```python
from build123d import *

# Parameters (mm, degrees)
SKETCH2_W           = 62.5
SKETCH2_H           = 62.5
CUT_EXTRUDE1_DEPTH  = 50
BOSS_EXTRUDE1_REACH = 166.055
SKETCH3_R           = 10
FILLET1_R           = 25


with BuildPart() as part:
    # Sketch1 → Revolve1 (revolve)
    with BuildSketch(Plane.XY, mode=Mode.PRIVATE) as revolve1_sk:
        Polygon((0, 0), (0, 100), (-75, 100), (-75, 68.75), (-67.5, 68.75), (-67.5, 61.25), (-75, 61.25), (-75, 53.75), (-67.5, 53.75), (-67.5, 46.25), (-75, 46.25), (-75, 38.75), (-67.5, 38.75), (-67.5, 31.25), (-75, 31.25), (-75, 0), align=None)
    revolve(revolve1_sk.sketch.rotate(Axis((0, 0, 0), (0, 1, 0)), 180), axis=Axis((0, 0, 0), (0, 1, 0)))

    # Sketch2 → Cut-Extrude1 (cut)
    with BuildSketch(Plane.XZ):
        Rectangle(SKETCH2_W, SKETCH2_H)
    extrude(amount=-CUT_EXTRUDE1_DEPTH, mode=Mode.SUBTRACT)

    # Sketch3 → Boss-Extrude1 (add, up to next)
    with BuildSketch(Plane.ZY.offset(-31.25), mode=Mode.PRIVATE) as boss_extrude1_sk1:
        with Locations(Location((0, 25, 0), (0, 0, 180))):
            Circle(SKETCH3_R)
    boss_extrude1_tool1 = extrude(boss_extrude1_sk1.sketch, amount=BOSS_EXTRUDE1_REACH, mode=Mode.PRIVATE) - part.part
    add(boss_extrude1_tool1.solids().sort_by_distance((31.25, 25, 0))[0])

    # Fillet1
    fillet1_edges = [part.edges().sort_by_distance(p)[0] for p in [
        (0, 50, -31.25),
        (0, 50, 31.25),
    ]]
    fillet(fillet1_edges, radius=FILLET1_R)


solid = part.part
```
Geometry check sheet. Reference: the model listing, model coordinates, mm. A direction names the side the tool comes from. Coordinates: 2 decimals unless noted, no trailing zeros. Write each loop counter-clockwise with the first axis right and the second up, starting at its lowest first coordinate (ties: lowest second). Pieces come first, ordered by that corner, then holes. Notation, with made-up numbers: M 37,45.5 L 90,45.5 A10 ccw 90,51.5 Z; hole C 85.25,-12.75 d4. An arc over 180 degrees is marked long. Use one line per item in the form item = value. Start each with the question number.
1) Go/stop test with flat-tipped pins: pin 1 Ø1.5 at (y, z) = (29.5, -54) entering from +X; pin 2 Ø10 at (x, y) = (-35.5, 32) entering from +Z; pin 3 Ø2 at (x, y) = (-55.5, 46.5) entering from +Z; pin 4 Ø25 at (y, z) = (17.5, 8.5) entering from +X. Record where each tip stops, or that it passes through.
2) Set-up check for faces 5 (the cylindrical face through (34.608, 15.406, 66.538)), 6 (the flat face through (0, 12, 31.25)), 7 (the flat face through (-67, 53.75, -11)): record each of +Z, -Z, +X, -X, +Y, -Y from which the full face is reachable in a straight line by a thin tool's end or side.
3) Section check C-C on y = 78. Enter the section's corners in (x, z), and give its area (3 significant figures).
4) Thickness scan on probe 1 along Y at (x, z) = (-14, 66.5); probe 2 along Z at (x, y) = (22.5, 23.5); probe 3 along X at (y, z) = (43, -1). Record the ranges inside material, lowest first. Write a range as from..to.
5) Release check for a two-part mould opening along Y. For faces 1 (the flat face through (-1, 0, 32)), 2 (the flat face through (1, 100, -1)), 3 (the flat face through (-31.25, 14, 0)), 4 (the flat face through (67, 46.25, -11)) record: pulls with the +Y half, pulls with the -Y half, needs draft (parallel to the pull), parting line crosses it, or undercut.
6) Section check A-A on y = 9. Enter the section's corners in (x, z).
7) Section check D-D on x = -52. Enter the section's corners in (y, z).
Responses:
q1.pin_1 = 52.82
q1.pin_2 = 68.49
q1.pin_3 = 51.49
q1.pin_4 = 75
q2.face_5 = +Y, -Y
q2.face_6 = -Y
q2.face_7 = none
q3.outline = C 0,0 d150
q3.area = 17,700 mm2
q4.probe_1 = 0..31.25, 38.75..46.25, 53.75..61.25, 68.75..100
q4.probe_2 = -71.55..-31.25, -9.89..9.89, 31.25..71.55
q4.probe_3 = -74.99..-31.25, 31.25..74.99
q5.face_1 = pulls with the -Y half
q5.face_2 = pulls with the +Y half
q5.face_3 = undercut
q5.face_4 = undercut
q6.outline = C 0,0 d150; hole M -31.25,-31.25 L 31.25,-31.25 L 31.25,31.25 L -31.25,31.25 Z
q7.outline = M 0,-54.05 L 31.25,-54.05 L 31.25,-43.04 L 38.75,-43.04 L 38.75,-54.05 L 46.25,-54.05 L 46.25,-43.04 L 53.75,-43.04 L 53.75,-54.05 L 61.25,-54.05 L 61.25,-43.04 L 68.75,-43.04 L 68.75,-54.05 L 100,-54.05 L 100,54.05 L 68.75,54.05 L 68.75,43.04 L 61.25,43.04 L 61.25,54.05 L 53.75,54.05 L 53.75,43.04 L 46.25,43.04 L 46.25,54.05 L 38.75,54.05 L 38.75,43.04 L 31.25,43.04 L 31.25,54.05 L 0,54.05 Z
